The listing builds one solid part. Answer for the finished solid, in the listing's coordinates (mm). A direction names the side the tool comes from. Round coordinates to 2 decimals unless told otherwise and drop trailing zeros. Write each loop counter-clockwise with the first axis right and the second up, starting at its lowest first coordinate (ties: lowest second). Pieces come first, ordered by that corner, then holes. Notation, with made-up numbers: (-35, -3.5) - (-22, -3.5) arc R15 cw to (-22, 9.5) - close; hole circle Ø4 at (-13.5, -28). An arc over 180 degrees is marked (long way). Use a Markdown table: item, result. Add a question column.
1) A cutting plane is placed at D-D (x = -9). Give the vertices of the cut face in (y, z).
2) Determine the mould class of faces 4 (the flat face through (5, 47, -44)), 5 (the cylindrical face through (-87.468, 27.002, 2.535)), 6 (the flat face through (-54, 48, 5)) for opening direction X: +X half, -X half, draft (parallel to the pull), parting line (faces both ways), or undercut.
3) Find the intervals of material crossed by probe 1 along X at (y, z) = (1.8, 55); probe 2 along Y at (x, z) = (-95.5, 1.5); probe 3 along Z at (x, y) = (-100, 1), in increasing order. Write a range as from..to.
4) A cutting plane is placed at A-A (x = -80). Give the vertices of the cut face in (y, z).
5) A tool of negligible diameter and unlimited length cuts with its end or side. For faces 1 (the flat face through (-80, 31.35, 3)), 2 (the cylindrical face through (2.15, 47.04, 1.99)), 3 (the flat face through (0, 39, -44)), from which of +Z, -Z, +X, -X, +Y, -Y can it reach the whole face along a straight path? Write none if from no direction.
6) A cutting plane is placed at C-C (y = 62). Give the vertices of the cut face in (x, z), then the cut area to 3 significant figures.
7) A cutting plane is placed at B-B (z = -33). Give the vertices of the cut face in (x, y), then the cut area to 3 significant figures.
8) Each of these flat-tipped pins is pushed along its axis until it touches: P1, Ø4, axis at x = -78.5, y = 24.5, coming from the -Z side; P2, Ø6, axis at x = -33.5, y = 70.5, coming from the +Z side; P3, Ø2.5, axis at x = -100, z = 55, coming from the +Y side; P4, Ø6, axis at y = 71.5, z = -4.5, coming from the -X side. Where does it stop, or does it pass through?
```python
from build123d import *

# Parameters (mm, degrees)
BOSS_EXTRUDE1_DEPTH = 20
SKETCH2_W           = 5
SKETCH2_H           = 85
BOSS_EXTRUDE2_DEPTH = 60
SKETCH3_R           = 15
CUT_EXTRUDE1_DEPTH  = 100
SKETCH4_R           = 1.25
CUT_EXTRUDE2_DEPTH  = 100
SKETCH7_W           = 110
SKETCH7_H           = 5
BOSS_EXTRUDE6_DEPTH = 60
FILLET3_R           = 5
SKETCH8_W           = 25
SKETCH8_H           = 145
SKETCH8_H_2         = 25
SKETCH8_W_2         = 185
CUT_EXTRUDE3_DEPTH  = 100
SKETCH9_R           = 1.65
CUT_EXTRUDE4_DEPTH  = 100
SKETCH10_W          = 75
SKETCH10_H          = 55
SKETCH10_W_2        = 110
SKETCH10_H_2        = 90
CUT_EXTRUDE5_DEPTH  = 15
FILLET4_R           = 10
SKETCH11_W          = 20
SKETCH11_H          = 5
CUT_EXTRUDE6_DEPTH  = 6
FILLET5_R           = 5
SKETCH12_R          = 15
SKETCH12_R_2        = 1.25
CUT_EXTRUDE7_DEPTH  = 10
SKETCH13_W          = 20
SKETCH13_H          = 145
CUT_EXTRUDE8_DEPTH  = 10


with BuildPart() as part:
    # Sketch1 → Boss-Extrude1 (new body)
    with BuildSketch(Plane(origin=(0, 0, 0), x_dir=(1, 0, 0), z_dir=(0, 1, 0))):
        Polygon((105, 85), (0, 85), (0, 0), (-105, 0), (-105, -85), (105, -85), align=None)
    extrude(amount=BOSS_EXTRUDE1_DEPTH)

    # Sketch2 → Boss-Extrude2 (add)
    with BuildSketch(Plane(origin=(0, 20, 0), x_dir=(1, 0, 0), z_dir=(0, 1, 0))):
        with Locations((2.5, 42.5)):
            Rectangle(SKETCH2_W, SKETCH2_H)
    extrude(amount=BOSS_EXTRUDE2_DEPTH)

    # Sketch3 → Cut-Extrude1 (cut)
    with BuildSketch(Plane.ZY):
        with Locations((-60, 58.85)):
            Circle(SKETCH3_R)
    extrude(amount=-CUT_EXTRUDE1_DEPTH, mode=Mode.SUBTRACT)

    # Sketch4 → Cut-Extrude2 (cut)
    with BuildSketch(Plane.ZY):
        with Locations((-75.5, 74.35)):
            Circle(SKETCH4_R)
        with Locations((-44.5, 74.35)):
            Circle(SKETCH4_R)
        with Locations((-75.5, 43.35)):
            Circle(SKETCH4_R)
        with Locations((-44.5, 43.35)):
            Circle(SKETCH4_R)
    extrude(amount=-CUT_EXTRUDE2_DEPTH, mode=Mode.SUBTRACT)

    # Sketch7 → Boss-Extrude6 (add)
    with BuildSketch(Plane(origin=(0, 20, 0), x_dir=(1, 0, 0), z_dir=(0, 1, 0))):
        with Locations((-50, -2.5)):
            Rectangle(SKETCH7_W, SKETCH7_H)
    extrude(amount=BOSS_EXTRUDE6_DEPTH)

    # Fillet3
    fillet3_edges = [part.edges().sort_by_distance(p)[0] for p in [
        (0, 40, 0),
    ]]
    fillet(fillet3_edges, radius=FILLET3_R)

    # Sketch8 → Cut-Extrude3 (cut)
    with BuildSketch(Plane(origin=(0, 20, 0), x_dir=(1, 0, 0), z_dir=(0, 1, 0))):
        with Locations((92.5, 12.5)):
            Rectangle(SKETCH8_W, SKETCH8_H)
        with Locations((92.5, -72.5)):
            Rectangle(SKETCH8_W, SKETCH8_H_2)
        with Locations((-12.5, -72.5)):
            Rectangle(SKETCH8_W_2, SKETCH8_H_2)
    extrude(amount=-CUT_EXTRUDE3_DEPTH, mode=Mode.SUBTRACT)

    # Sketch9 → Cut-Extrude4 (cut)
    with BuildSketch(Plane(origin=(0, 20, 0), x_dir=(1, 0, 0), z_dir=(0, 1, 0))):
        with Locations(Location((55, 80, 0), (0, 0, 270))):
            Circle(SKETCH9_R)
        with Locations(Location((55, -55, 0), (0, 0, 270))):
            Circle(SKETCH9_R)
        with Locations(Location((-100, -55, 0), (0, 0, 270))):
            Circle(SKETCH9_R)
    extrude(amount=-CUT_EXTRUDE4_DEPTH, mode=Mode.SUBTRACT)

    # Sketch10 → Cut-Extrude5 (cut)
    with BuildSketch(Plane(origin=(0, 20, 0), x_dir=(1, 0, 0), z_dir=(0, 1, 0))):
        with Locations((42.5, -32.5)):
            Rectangle(SKETCH10_W, SKETCH10_H)
        with Locations((-50, -32.5)):
            Rectangle(SKETCH10_W_2, SKETCH10_H)
        with Locations((42.5, 40)):
            Rectangle(SKETCH10_W, SKETCH10_H_2)
    extrude(amount=-CUT_EXTRUDE5_DEPTH, mode=Mode.SUBTRACT)

    # Fillet4
    fillet4_edges = [part.edges().sort_by_distance(p)[0] for p in [
        (5, 5, -40),
        (-50, 5, 5),
        (5, 42.5, 5),
    ]]
    fillet(fillet4_edges, radius=FILLET4_R)

    # Sketch11 → Cut-Extrude6 (cut)
    with BuildSketch(Plane.XY.offset(5)):
        with Locations((-80, 28.85)):
            Rectangle(SKETCH11_W, SKETCH11_H)
    extrude(amount=-CUT_EXTRUDE6_DEPTH, mode=Mode.SUBTRACT)

    # Fillet5
    # the kernel refuses this fillet: 5 mm, written as the material it adds along each edge
    with BuildSketch(Plane(origin=(-90, 26.35, 5), x_dir=(0, 1, 0), z_dir=(0, 0, -1))) as fillet5_piece_1:
        with BuildLine():
            CenterArc((FILLET5_R, FILLET5_R), FILLET5_R, 180, 90)
            Line((0, FILLET5_R), (0, 0))
            Line((0, 0), (FILLET5_R, 0))
        make_face()
    extrude(amount=5)
    with BuildSketch(Plane(origin=(-90, 31.35, 5), x_dir=(0, -1, 0), z_dir=(0, 0, -1)), Plane(origin=(-70, 31.35, 5), x_dir=(-1, 0, 0), z_dir=(0, 0, -1)), Plane(origin=(-70, 26.35, 5), x_dir=(0, 1, 0), z_dir=(0, 0, -1))) as fillet5_piece_2:
        with BuildLine():
            CenterArc((FILLET5_R, -FILLET5_R), FILLET5_R, 90, 90)
            Line((0, -FILLET5_R), (0, 0))
            Line((0, 0), (FILLET5_R, 0))
        make_face()
    extrude(amount=5)

    # Sketch12 → Cut-Extrude7 (cut)
    with BuildSketch(Plane(origin=(0, 0, 0), x_dir=(-1, 0, 0), z_dir=(0, 0, -1))):
        with Locations((80, 58.85)):
            Circle(SKETCH12_R)
        with Locations((95.5, 74.35)):
            Circle(SKETCH12_R_2)
        with Locations((64.5, 74.35)):
            Circle(SKETCH12_R_2)
        with Locations((64.5, 43.35)):
            Circle(SKETCH12_R_2)
        with Locations((95.5, 43.35)):
            Circle(SKETCH12_R_2)
    extrude(amount=-CUT_EXTRUDE7_DEPTH, mode=Mode.SUBTRACT)

    # Sketch13 → Cut-Extrude8 (cut)
    with BuildSketch(Plane(origin=(0, 5, 0), x_dir=(1, 0, 0), z_dir=(0, 1, 0))):
        with Locations((70, 12.5)):
            Rectangle(SKETCH13_W, SKETCH13_H)
    extrude(amount=-CUT_EXTRUDE8_DEPTH, mode=Mode.SUBTRACT)


solid = part.part
```
Entries:
| question | item | result |
|---|---|---|
| 1 | outline | (0, 0) - (80, 0) - (80, 5) - (15, 5) arc R10 cw to (5, 15) - (5, 60) - (0, 60) - close |
| 2 | face 4 | +X half |
| 2 | face 5 | undercut |
| 2 | face 6 | draft |
| 3 | probe 1 | x = -105..-101.65, -98.35..53.35, 56.65..60 |
| 3 | probe 2 | y = 0..42.1, 44.6..73.1, 75.6..80 |
| 3 | probe 3 | z = 0..53.35, 56.65..60 |
| 4 | outline | (0, 0) - (26.35, 0) - (26.35, 5) - (15, 5) arc R10 cw to (5, 15) - (5, 60) - (0, 60) - close; (31.35, 0) - (43.85, 0) - (43.85, 5) - (31.35, 5) - close; (73.85, 0) - (80, 0) - (80, 5) - (73.85, 5) - close |
| 5 | face 1 | +Z, -Z |
| 5 | face 2 | +Z, +X, +Y |
| 5 | face 3 | -Z, -X, +Y, -Y |
| 6 | outline | (-105, 0) - (-94.67, 0) - (-94.67, 5) - (-105, 5) - close; (-65.33, 0) - (-5, 0) arc R5 cw to (0, -5) - (0, -45.33) - (5, -45.33) - (5, -5) arc R10 ccw to (-5, 5) - (-65.33, 5) - close; (0, -85) - (5, -85) - (5, -74.67) - (0, -74.67) - close |
| 6 | area | 666 mm² |
| 7 | outline | (0, 0) - (60, 0) - (60, 5) - (15, 5) arc R10 cw to (5, 15) - (5, 80) - (0, 80) - close |
| 7 | area | 696 mm² |
| 8 | P1 | stops at z = 0 |
| 8 | P2 | stops at z = 5 |
| 8 | P3 | passes through |
| 8 | P4 | stops at x = -1.43 |
